Read the model definition and answer for the solid it produces. Units are mm, in the model's axes. A direction names the side the tool comes from. Give positions to 0.01 mm unless a question says otherwise; leave off trailing zeros. Loops run counter-clockwise (first coordinate to the right, second up) from the corner with the lowest first, then second, coordinate; pieces in that order, holes last. Notation, with made-up numbers: (21.25, 38.25) - (68.25, 38.25) arc R18 cw to (68.25, 69.25) - close; hole circle Ø3 at (-24.5, 15.5). An arc over 180 degrees is marked (long way). Use a Markdown table: item, result. Add a question column.
Item 1: For a pull along Y with two mould halves and no side action, classify faces 4 (the face through (-14, 42.55, -20)), 5 (the face through (-34.59, -29.06, -22.75)), 6 (the face through (-49.4, 21.64, -19.57)) as +Y half, -Y half, draft (parallel to the pull), parting line (faces both ways), or undercut.
Item 2: Each of these flat-tipped pins is pushed along its axis until it touches: P1, Ø6, axis at x = -23.5, y = 4, coming from the +Z side; P2, Ø13, axis at x = -32, y = 32.43, coming from the -Z side; P3, Ø1.2, axis at x = -2.5, y = 30, coming from the -Z side; P4, Ø6, axis at y = 13.5, z = -12.5, coming from the +X side. Where does it stop, or does it pass through?
Item 3: A cutting plane is placed at B-B (x = -32). Give the number of separate pieces and of enclosed holes in the cut face, plus the area to 4 significant figures.
Item 4: A cutting plane is placed at A-A (y = -32.43). Determine the outline of the cut face in (x, z).
Item 5: A cutting plane is placed at D-D (x = -1). Determine the outline of the cut face in (y, z), plus the area to 3 significant figures.
Item 6: Consider probe 1 along X at (y, z) = (-11.43, -23.55); probe 2 along Y at (x, z) = (-31, -23); probe 3 along Y at (x, z) = (-32, -19.65). Determine where each line is inside the solid, lowest interval first. Write a range as [from, to].
Item 7: Which of the six approach directions +Z, -Z, +X, -X, +Y, -Y give full straight-line access (tool end or side, diameter ignored) to faces 1 (the face through (-35.966, -10.909, -23.507)), 2 (the face through (-10, 22, -15)), 3 (the face through (-8, 0, -18))?
Item 8: A cutting plane is placed at C-C (y = -23). Determine the outline of the cut face in (x, z), plus the area to 3 significant figures.
Autodesk Inventor part; units mm, degrees
ref_plane "side_2a_XY" through (-32, -21.925, -19) normal (0, 0, 1) x (1, 0, 0)
ref_plane "side_2a_YZ" through (-32, -21.925, -19) normal (1, 0, 0) x (0, 1, 0)
ref_plane "side_2a_ZX" through (-32, -21.925, -19) normal (0, 1, 0) x (0, 0, 1)
sketch "Skizze_34" plane through (0, 0, 0) normal (0, 1, 0) x (1, 0, 0)
  circle A0 centre (0, 12) radius 10
extrude "Extrusion1" add sketch "Skizze_34" along normal mid plane 2.5
sketch "Skizze_35" plane through (0, 0, 0) normal (0, 1, 0) x (1, 0, 0)
  circle A0 centre (0, 12) radius 6
extrude "Extrusion2" add sketch "Skizze_35" along normal mid plane 85.5
sketch "Skizze_36" plane through (0, -1.3, 0) normal (0, 1, 0) x (1, 0, 0)
  line L0 (-50, 24) -> (-50, 21)
  arc A0 (-50, 21) -> (-48, 19) centre (-48, 21) ccw
  line L1 (-48, 19) -> (-12, 19)
  arc A1 (-10, 17) -> (-12, 19) centre (-12, 17) ccw
  line L2 (-10, 17) -> (-10, 12)
  arc A2 (-10, 12) -> (0, 22) centre (0, 12) ccw
  line L3 (0, 22) -> (-4, 22)
  arc A3 (-5.8856, 23.3333) -> (-4, 22) centre (-4, 24) ccw
  arc A4 (-5.8856, 23.3333) -> (-6.8284, 24) centre (-6.8284, 23) ccw
  line L4 (-6.8284, 24) -> (-50, 24)
  circle A5 centre (0, 12) radius 6
extrude "Extrusion3" add sketch "Skizze_36" against normal blind 41.25
sketch "Skizze_37" plane through (0, 1.3, 0) normal (0, 1, 0) x (1, 0, 0)
  line L0 (-50, 24) -> (-50, 21)
  arc A0 (-50, 21) -> (-48, 19) centre (-48, 21) ccw
  line L1 (-48, 19) -> (-12, 19)
  arc A1 (-10, 17) -> (-12, 19) centre (-12, 17) ccw
  line L2 (-10, 17) -> (-10, 12)
  arc A2 (-10, 12) -> (0, 22) centre (0, 12) ccw
  line L3 (0, 22) -> (-4, 22)
  arc A3 (-5.8856, 23.3333) -> (-4, 22) centre (-4, 24) ccw
  arc A4 (-5.8856, 23.3333) -> (-6.8284, 24) centre (-6.8284, 23) ccw
  line L4 (-6.8284, 24) -> (-50, 24)
  circle A5 centre (0, 12) radius 6
extrude "Extrusion4" add sketch "Skizze_37" along normal blind 41.25
sketch "Sketch5" plane through (-6.8284, 1.3, -24) normal (0, 0, -1) x (-1, 0, 0)
  point P0 (25.1716, 10.13)
hole "Drilling 1" at (-32, 11.43, -24) direction (0, 0, 1) diameter 8 depth 5 countersink diameter 16 countersink angle 90
sketch "Sketch6" plane through (-6.8284, 1.3, -24) normal (0, 0, -1) x (-1, 0, 0)
  point P0 (25.1716, 31.13)
hole "Drilling 2" at (-32, 32.43, -24) direction (0, 0, 1) diameter 8 depth 5 countersink diameter 16 countersink angle 90
sketch "Sketch7" plane through (-48, -1.3, -19) normal (0, 0, 1) x (1, 0, 0)
  point P0 (16, -10.13)
hole "Drilling 3" at (-32, -11.43, -19) direction (0, 0, -1) diameter 8 depth 5 countersink diameter 16 countersink angle 90
sketch "Sketch8" plane through (-48, -1.3, -19) normal (0, 0, 1) x (1, 0, 0)
  point P0 (16, -31.13)
hole "Drilling 4" at (-32, -32.43, -19) direction (0, 0, -1) diameter 8 depth 5 countersink diameter 16 countersink angle 90
ref_plane "side_2a_XY" through (-32, -21.925, -19) normal (0, 0, 1) x (1, 0, 0)
ref_plane "side_2a_YZ" through (-32, -21.925, -19) normal (1, 0, 0) x (0, 1, 0)
ref_plane "side_2a_ZX" through (-32, -21.925, -19) normal (0, 1, 0) x (0, 0, 1)
ref_plane "side_2b_XY" through (-32, -21.925, -24) normal (0, 0, -1) x (1, 0, 0)
ref_plane "side_2b_YZ" through (-32, -21.925, -24) normal (1, 0, 0) x (0, -1, 0)
ref_plane "side_2b_ZX" through (-32, -21.925, -24) normal (0, -1, 0) x (0, 0, -1)
ref_plane "side_1b_XY" through (-32, 21.925, -19) normal (0, 0, 1) x (1, 0, 0)
ref_plane "side_1b_YZ" through (-32, 21.925, -19) normal (1, 0, 0) x (0, 1, 0)
ref_plane "side_1b_ZX" through (-32, 21.925, -19) normal (0, 1, 0) x (0, 0, 1)
ref_plane "side_3b_XY" through (-32, 21.925, -19) normal (0, 0, 1) x (1, 0, 0)
ref_plane "side_3b_YZ" through (-32, 21.925, -19) normal (1, 0, 0) x (0, 1, 0)
ref_plane "side_3b_ZX" through (-32, 21.925, -19) normal (0, 1, 0) x (0, 0, 1)
ref_plane "side_1a_XY" through (-32, 21.925, -24) normal (0, 0, -1) x (1, 0, 0)
ref_plane "side_1a_YZ" through (-32, 21.925, -24) normal (1, 0, 0) x (0, -1, 0)
ref_plane "side_1a_ZX" through (-32, 21.925, -24) normal (0, -1, 0) x (0, 0, -1)
ref_plane "side_3a_XY" through (-32, 21.925, -24) normal (0, 0, -1) x (1, 0, 0)
ref_plane "side_3a_YZ" through (-32, 21.925, -24) normal (1, 0, 0) x (0, -1, 0)
ref_plane "side_3a_ZX" through (-32, 21.925, -24) normal (0, -1, 0) x (0, 0, -1)
properties part number "MayTec 1.62.842032085_Alu hinges, heavy, type 20 PG 40 (0)"
Geometry says:
| question | item | result |
|---|---|---|
| 1 | face 4 | +Y half |
| 1 | face 5 | undercut |
| 1 | face 6 | draft |
| 2 | P1 | z = -19 |
| 2 | P2 | z = -22.5 |
| 2 | P3 | z = -22 |
| 2 | P4 | x = 10 |
| 3 | separate pieces | 6 |
| 3 | enclosed holes | 0 |
| 3 | area | 188.5 mm² |
| 4 | outline | (-50, -24) - (-36, -24) - (-36, -23) - (-40, -19) - (-48, -19) arc R2 ccw to (-50, -21) - close; (-28, -24) - (-6.83, -24) arc R1 ccw to (-5.89, -23.33) arc R2 cw to (-4, -22) - (0, -22) arc R10 ccw (long way) to (-10, -12) - (-10, -17) arc R2 cw to (-12, -19) - (-24, -19) - (-28, -23) - close |
| 5 | outline | (-42.75, -17.92) - (-42.55, -17.92) - (-42.55, -22) - (-1.3, -22) - (-1.3, -17.92) - (-1.25, -17.92) - (-1.25, -21.95) - (1.25, -21.95) - (1.25, -17.92) - (1.3, -17.92) - (1.3, -22) - (42.55, -22) - (42.55, -17.92) - (42.75, -17.92) - (42.75, -6.08) - (42.55, -6.08) - (42.55, -2.05) - (1.3, -2.05) - (1.3, -6.08) - (1.25, -6.08) - (1.25, -2.05) - (-1.25, -2.05) - (-1.25, -6.08) - (-1.3, -6.08) - (-1.3, -2.05) - (-42.55, -2.05) - (-42.55, -6.08) - (-42.75, -6.08) - close |
| 5 | area | 1,700 mm² |
| 6 | probe 1 | [-50, -36], [-28, -5.99] |
| 6 | probe 2 | [-42.55, -36.3], [-28.56, -15.3], [-7.56, -1.3], [1.3, 4.5], [18.36, 25.5], [39.36, 42.55] |
| 6 | probe 3 | [-42.55, -39.78], [-25.08, -18.78], [-4.08, -1.3], [1.3, 7.43], [15.43, 28.43], [36.43, 42.55] |
| 7 | face 1 | +Z, -Z |
| 7 | face 2 | +Z, -X, +Y, -Y |
| 7 | face 3 | none |
| 8 | outline | (-50, -24) - (-6.83, -24) arc R1 ccw to (-5.89, -23.33) arc R2 cw to (-4, -22) - (0, -22) arc R10 ccw (long way) to (-10, -12) - (-10, -17) arc R2 cw to (-12, -19) - (-48, -19) arc R2 ccw to (-50, -21) - close |
| 8 | area | 544 mm² |
